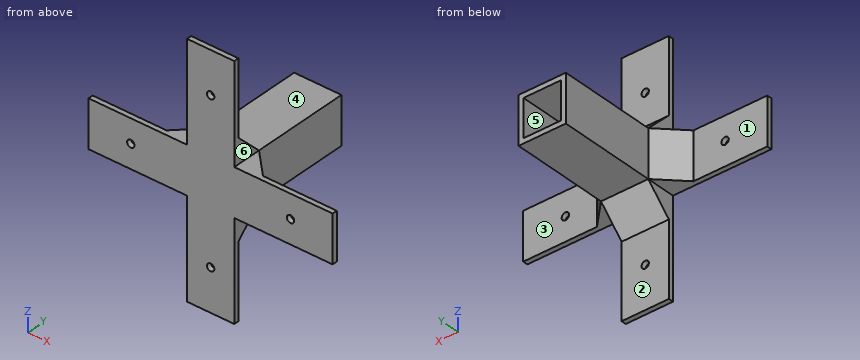
from build123d import *

# Parameters (mm, degrees)
SKETCH1_W           = 19.2
SKETCH1_H           = 19.2
SKETCH1_W_2         = 15.2
SKETCH1_H_2         = 15.2
EXTRUDE_THIN1_DEPTH = 50
BOSS_EXTRUDE1_DEPTH = 2
CHAMFER1_SIZE       = 10
CHAMFER2_SIZE       = 10
CHAMFER3_SIZE       = 10
CHAMFER4_SIZE       = 10
SKETCH6_R           = 1.5
CUT_EXTRUDE1_DEPTH  = 87.141279303


# Some blends are built 0.0001 mm under size
with BuildPart() as part:
    # Sketch1 → Extrude-Thin1 (new body)
    with BuildSketch(Plane(origin=(0, 0, 0), x_dir=(1, 0, 0), z_dir=(0, 1, 0))):
        Rectangle(SKETCH1_W, SKETCH1_H)
        Rectangle(SKETCH1_W_2, SKETCH1_H_2, mode=Mode.SUBTRACT)
    extrude(amount=EXTRUDE_THIN1_DEPTH)

    # Sketch2 → Boss-Extrude1 (add)
    with BuildSketch(Plane(origin=(0, 0, 0), x_dir=(1, 0, 0), z_dir=(0, 1, 0))):
        Polygon((9.6, 9.6), (49.6, 9.6), (49.6, -9.6), (9.6, -9.6), (9.6, -49.6), (-9.6, -49.6), (-9.6, -9.6), (-49.6, -9.6), (-49.6, 9.6), (-9.6, 9.6), (-9.6, 49.6), (9.6, 49.6), align=None)
    extrude(amount=-BOSS_EXTRUDE1_DEPTH)

    # Chamfer1
    # the kernel refuses this chamfer: 10 mm, written as the material it adds along each edge
    with BuildSketch(Plane(origin=(-9.6, 0, 9.6), x_dir=(0, 1, 0), z_dir=(0, 0, -1))) as chamfer1_piece_1:
        Polygon((CHAMFER1_SIZE, 0), (0, -CHAMFER1_SIZE), (0, 0), align=None)
    extrude(amount=19.2)

    # Chamfer2
    # the kernel refuses this chamfer: 10 mm, written as the material it adds along each edge
    with BuildSketch(Plane(origin=(-9.6, 0, -9.6), x_dir=(0, 1, 0), z_dir=(1, 0, 0))) as chamfer2_piece_1:
        Polygon((CHAMFER2_SIZE, 0), (0, -CHAMFER2_SIZE), (0, 0), align=None)
    extrude(amount=19.2)

    # Chamfer3
    # the kernel refuses this chamfer: 10 mm, written as the material it adds along each edge
    with BuildSketch(Plane(origin=(9.6, 0, -9.6), x_dir=(0, 1, 0), z_dir=(0, 0, 1))) as chamfer3_piece_1:
        Polygon((CHAMFER3_SIZE, 0), (0, -CHAMFER3_SIZE), (0, 0), align=None)
    extrude(amount=19.2)

    # Chamfer4
    chamfer4_edges = [part.edges().sort_by_distance(p)[0] for p in [
        (0, 0, 9.6),
    ]]
    chamfer(chamfer4_edges, length=CHAMFER4_SIZE - 0.0001)  # a hair under: the kernel refuses the full size

    # Sketch6 → Cut-Extrude1 (cut, through all)
    with BuildSketch(Plane(origin=(0, 0, 0), x_dir=(1, 0, 0), z_dir=(0, 1, 0))):
        with Locations(Location((0, 32.455385939, 0), (0, 0, 270))):
            Circle(SKETCH6_R)
        with Locations(Location((32.455385939, 0, 0), (0, 0, 270))):
            Circle(SKETCH6_R)
        with Locations(Location((0, -32.455385939, 0), (0, 0, 270))):
            Circle(SKETCH6_R)
        with Locations(Location((-32.455385939, 0, 0), (0, 0, 270))):
            Circle(SKETCH6_R)
    extrude(amount=-CUT_EXTRUDE1_DEPTH, mode=Mode.SUBTRACT)


solid = part.part
Can you work these out from the model? Positions are in its coordinate system, mm. Face numbers are marked on the shaded views. A direction names the side the tool comes from. Give positions to 0.01 mm unless a question says otherwise; leave off trailing zeros. Write each loop counter-clockwise with the first axis right and the second up, starting at its lowest first coordinate (ties: lowest second). Pieces come first, ordered by that corner, then holes. Notation, with made-up numbers: (4, -17.5) -> (22, -17.5) arc R31 cw to (22, 8.5) -> close; hole circle Ø2 at (67.5, 19). An arc over 180 degrees is marked (long way). Answer as a JSON object with one key per item and string values. Group by question number.
Item 1: Suppose I cut it at B-B (z = 0). Please give me the cut outline in (x, y).
Item 2: Suppose I cut it at A-A (x = 0). Please give me the cut outline in (y, z), plus the area to 3 significant figures.
Item 3: We'd pull the mould along Z, two halves only. Please class the marked faces 4, 5 and 6: +Z half, -Z half, draft (parallel to the pull), parting line (faces both ways), or undercut.
Item 4: For the marked faces 1, 2 and 3, which set-ups out of +Z, -Z, +X, -X, +Y, -Y let a thin tool reach every point of the face, with its end or its side?
Item 5: I'm going to push flat-ended pins straight in: P1, Ø21, axis at x = -2, z = -28.5, coming from the +Y side; P2, Ø9.5, axis at x = 1, z = 28, coming from the +Y side; P3, Ø5, axis at x = 9.5, y = 31, coming from the -Z side; P4, Ø5, axis at x = 0, z = 32.46, coming from the -Y side. Where does each tip first touch, or does it pass through?
Item 6: Suppose I cut it at D-D (x = 43.5). Please give me the cut outline in (y, z).
Item 7: Please list where these lines run through material, in increasing order: line 1 (X direction, y = 36.5, z = 3.5); line 2 (Y direction, x = 3, z = -31.5). Write a range as [from, to].
Item 8: Suppose I cut it at C-C (y = 19). Please give me the cut outline in (x, z), plus the area to 3 significant figures.
Findings:
{
 "1": {"outline": "(-49.6, -2) -> (-33.96, -2) -> (-33.96, 0) -> (-49.6, 0) -> close; (-30.96, -2) -> (30.96, -2) -> (30.96, 0) -> (19.6, 0) -> (9.6, 10) -> (9.6, 50) -> (7.6, 50) -> (7.6, 0) -> (-7.6, 0) -> (-7.6, 50) -> (-9.6, 50) -> (-9.6, 10) -> (-19.6, 0) -> (-30.96, 0) -> close; (33.96, -2) -> (49.6, -2) -> (49.6, 0) -> (33.96, 0) -> close"},
 "2": {"outline": "(-2, -49.6) -> (0, -49.6) -> (0, -33.96) -> (-2, -33.96) -> close; (-2, -30.96) -> (0, -30.96) -> (0, -19.6) -> (10, -9.6) -> (50, -9.6) -> (50, -7.6) -> (0, -7.6) -> (0, 7.6) -> (50, 7.6) -> (50, 9.6) -> (10, 9.6) -> (0, 19.6) -> (0, 30.96) -> (-2, 30.96) -> close; (-2, 33.96) -> (0, 33.96) -> (0, 49.6) -> (-2, 49.6) -> close", "area": "486 mm²"},
 "3": {"face 4": "+Z half", "face 5": "undercut", "face 6": "draft"},
 "4": {"face 1": "+Z, -Z, -X, +Y", "face 2": "-Z, +X, -X, +Y", "face 3": "+Z, -Z, +X, +Y"},
 "5": {"P1": "stops at y = 1.6", "P2": "stops at y = 0", "P3": "stops at z = -9.6", "P4": "stops at y = -2"},
 "6": {"outline": "(-2, -9.6) -> (0, -9.6) -> (0, 9.6) -> (-2, 9.6) -> close"},
 "7": {"line 1": "x = [-9.6, -7.6], [7.6, 9.6]", "line 2": "y = [-2, 0]"},
 "8": {"outline": "(-9.6, -9.6) -> (9.6, -9.6) -> (9.6, 9.6) -> (-9.6, 9.6) -> close; hole (-7.6, -7.6) -> (7.6, -7.6) -> (7.6, 7.6) -> (-7.6, 7.6) -> close", "area": "138 mm²"}
}
